Verification items for this drawing (mm, ordinates from the low corner). Coordinates: 2 decimals unless noted, no trailing zeros. Order: outer loops, then holes, each group sorted by start corner. A loop starts at its lowest first (then second) coordinate and runs counter-clockwise, first axis right, second up. Notation, with made-up numbers: M -31,39.5 L -20,39.5 A30 cw -20,62.5 Z; hole C -25,-14.75 d6. An arc over 180 degrees is marked long. Write item = value, one per line.
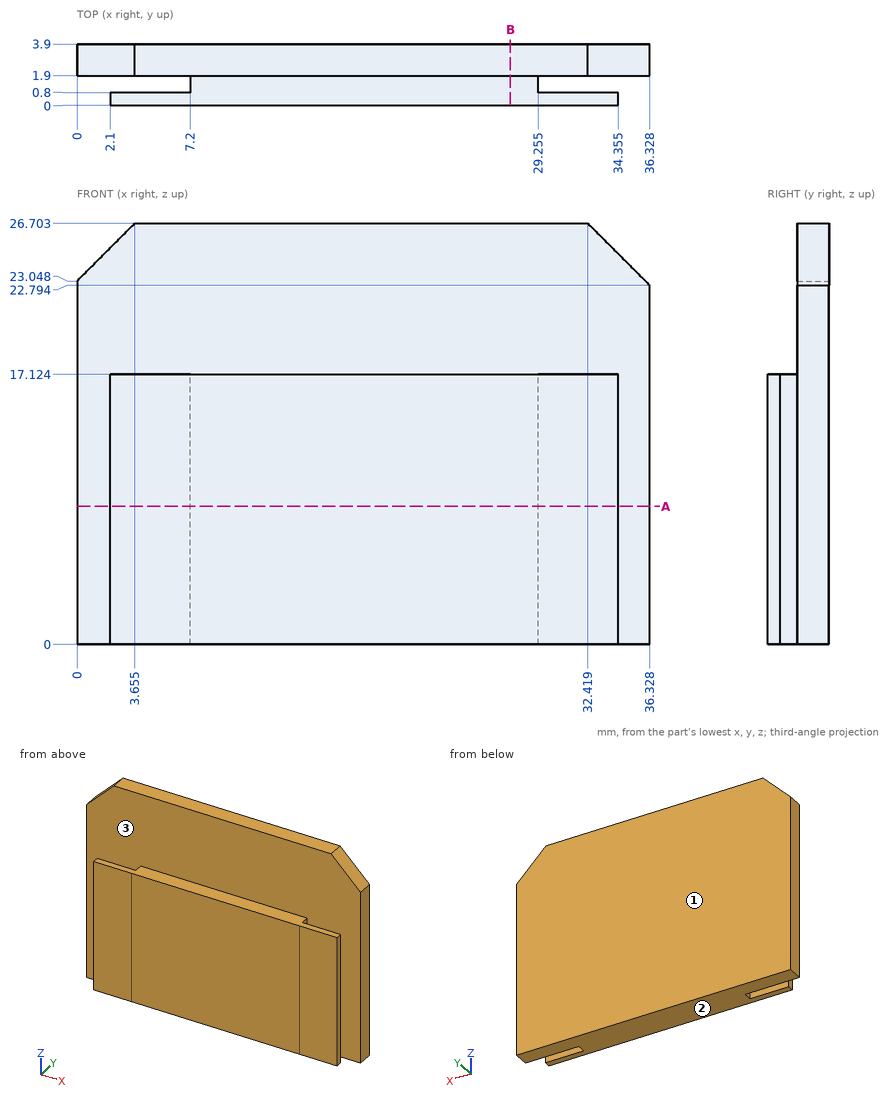
Item 1: Sectioned sample at A-A, the plane z = 8.75. Enter the section's corners in (x, y) (1 decimal), then the cut area to 3 significant figures.
Report:
outline = M 0,1.9 L 7.2,1.9 L 7.2,0.8 L 2.1,0.8 L 2.1,0 L 34.4,0 L 34.4,0.8 L 29.3,0.8 L 29.3,1.9 L 36.3,1.9 L 36.3,3.9 L 0,3.9 Z
area = 123 mm^2
Item 2: Scan lines: L1, parallel to Y at x = 31, z = 4; L2, parallel to Y at x = 34.5, z = 10.5; L3, parallel to Z at x = 24, y = 0.95. Record each from-to range of solid material in increasing order. Write a range as from..to.
Report:
L1 = 0..0.8, 1.9..3.9
L2 = 1.9..3.9
L3 = 0..17.12
Item 3: Gauge pin test, flat ends, axial feed: pin 1 (0.9 mm diameter, centred on x = 21.5, y = 1, fed in from +Z); pin 2 (0.6 mm diameter, centred on y = 0.5, z = 5.5, fed in from +X) (1 decimal); pin 3 (1.5 mm diameter, centred on y = 1, z = 14, fed in from -X). Record the tip position at first contact, or that the pin passes through.
Report:
pin_1 = 17.12
pin_2 = 34.4
pin_3 = 2.1
Item 4: Sectioned sample at B-B, the plane x = 27.5. Enter the section's corners in (y, z).
Report:
outline = M 0,0 L 3.9,0 L 3.9,26.7 L 1.9,26.7 L 1.9,17.12 L 0,17.12 Z
Item 5: Release check for a two-part mould opening along Y. For the marked faces 1, 2 and 3 record: pulls with the +Y half, pulls with the -Y half, needs draft (parallel to the pull), parting line crosses it, or undercut.
Report:
face_1 = pulls with the +Y half
face_2 = needs draft
face_3 = undercut
